Part model, mm, in its own coordinate system. A direction names the side the tool comes from. Round coordinates to 2 decimals unless told otherwise and drop trailing zeros. Write each loop counter-clockwise with the first axis right and the second up, starting at its lowest first coordinate (ties: lowest second). Pieces come first, ordered by that corner, then holes. Notation, with made-up numbers: M 63,23.25 L 78,23.25 A34 ccw 78,57.25 Z; hole C 70.5,36 d6. An arc over 180 degrees is marked long. Use a Markdown table: item, result. Add a question column.
1) Slice it at A-A on y = 16. Write the cut outline in (x, z), plus the area to 3 significant figures.
2) Drop flat-ended pins along their axis: P1, Ø0.9, axis at y = 17.5, z = 2, coming from the +X side; P2, Ø1.6, axis at x = -69.5, z = 2, coming from the -Y side; P3, Ø1.5, axis at y = 17.5, z = 1, coming from the -X side. Give the stop position or say it passes through.
3) Slice it at C-C on z = 1.8. Write the cut outline in (x, y), plus the area to 3 significant figures.
4) Which spindle directions (+Z, -Z, +X, -X, +Y, -Y) get a long thin tool onto all of the face, cutting with end or side? Do faces 4 (the face through (66.6, 21, 1)), 5 (the face through (66.6, -21, 1)), 6 (the face through (6, -20.5, 1)). Say none if no direction does.
5) Two-plate mould, pull along Y, no slides. Class faces 1 (the face through (-43.5, 0, 1)), 2 (the face through (65.17, -33.5, 1.48)), 3 (the face through (-66.6, 21, 1)): released by +Y, released by -Y, zero draft, split by the parting line, or undercut.
6) Slice it at D-D on x = 15.5. Write the cut outline in (y, z), plus the area to 3 significant figures.
7) Wall check: probe 1 along Y at (x, z) = (-40.7, 2.4); probe 2 along Y at (x, z) = (-19.5, 0.7); probe 3 along X at (y, z) = (28, 0.5). Give the ranges that are in metal, low to high.
8) Slice it at B-B on x = -40.7. Write the cut outline in (y, z).
```python
from build123d import *

# Parameters (mm, degrees)
ESQUISSE1_W                       = 101
ESQUISSE1_H                       = 41
BOSS_EXTRU_1_DEPTH                = 3
DIAM_TRE_DU_PER_AGE_3_0_3_1_D     = 3
DIAM_TRE_DU_PER_AGE_3_0_3_1_DEPTH = 3


with BuildPart() as part:
    # Esquisse1 → Boss.-Extru.1 (new body)
    with BuildSketch(Plane.XY):
        with BuildLine():
            Line((66.6, 30), (66.6, 12))
            ThreePointArc((66.6, 12), (67.185786438, 10.585786438), (68.6, 10))
            Line((68.6, 10), (70.6, 10))
            Line((70.6, 10), (70.6, -10))
            Line((70.6, -10), (68.6, -10))
            ThreePointArc((68.6, -10), (67.185786438, -10.585786438), (66.6, -12))
            Line((66.6, -12), (66.6, -30))
            ThreePointArc((66.6, -30), (65.135533906, -33.535533906), (61.6, -35))
            Line((61.6, -35), (-61.6, -35))
            ThreePointArc((-61.6, -35), (-65.135533906, -33.535533906), (-66.6, -30))
            Line((-66.6, -30), (-66.6, -12))
            ThreePointArc((-66.6, -12), (-67.185786438, -10.585786438), (-68.6, -10))
            Line((-68.6, -10), (-70.6, -10))
            Line((-70.6, -10), (-70.6, 10))
            Line((-70.6, 10), (-68.6, 10))
            ThreePointArc((-68.6, 10), (-67.185786438, 10.585786438), (-66.6, 12))
            Line((-66.6, 12), (-66.6, 30))
            ThreePointArc((-66.6, 30), (-65.135533906, 33.535533906), (-61.6, 35))
            Line((-61.6, 35), (61.6, 35))
            ThreePointArc((61.6, 35), (65.135533906, 33.535533906), (66.6, 30))
        make_face()
        with Locations((7, 0)):
            Rectangle(ESQUISSE1_W, ESQUISSE1_H, mode=Mode.SUBTRACT)
    extrude(amount=BOSS_EXTRU_1_DEPTH)

    # Diamètre du perçage Ø3.0 (3)1
    with Locations(Plane.XY.offset(3)):
        with Locations((-40.7, 27.7), (-40.7, -27.7), (54.7, -27.7), (54.7, 27.7)):
            Hole(DIAM_TRE_DU_PER_AGE_3_0_3_1_D / 2, depth=DIAM_TRE_DU_PER_AGE_3_0_3_1_DEPTH)


solid = part.part
```
Entries:
| question | item | result |
|---|---|---|
| 1 | outline | M -66.6,0 L -43.5,0 L -43.5,3 L -66.6,3 Z; M 57.5,0 L 66.6,0 L 66.6,3 L 57.5,3 Z |
| 1 | area | 96.6 mm^2 |
| 2 | P1 | stops at x = 66.6 |
| 2 | P2 | stops at y = -10 |
| 2 | P3 | stops at x = -66.6 |
| 3 | outline | M -70.6,-10 L -68.6,-10 A2 cw -66.6,-12 L -66.6,-30 A5 ccw -61.6,-35 L 61.6,-35 A5 ccw 66.6,-30 L 66.6,-12 A2 cw 68.6,-10 L 70.6,-10 L 70.6,10 L 68.6,10 A2 cw 66.6,12 L 66.6,30 A5 ccw 61.6,35 L -61.6,35 A5 ccw -66.6,30 L -66.6,12 A2 cw -68.6,10 L -70.6,10 Z; hole M -43.5,-20.5 L 57.5,-20.5 L 57.5,20.5 L -43.5,20.5 Z; hole C -40.7,-27.7 d3; hole C -40.7,27.7 d3; hole C 54.7,-27.7 d3; hole C 54.7,27.7 d3 |
| 3 | area | 5,300 mm^2 |
| 4 | face 4 | +Z, -Z, +X, +Y |
| 4 | face 5 | +Z, -Z, +X, -Y |
| 4 | face 6 | +Z, -Z |
| 5 | face 1 | undercut |
| 5 | face 2 | released by -Y |
| 5 | face 3 | zero draft |
| 6 | outline | M -35,0 L -20.5,0 L -20.5,3 L -35,3 Z; M 20.5,0 L 35,0 L 35,3 L 20.5,3 Z |
| 6 | area | 87.0 mm^2 |
| 7 | probe 1 | y = -35 to -29.2, -26.2 to -20.5, 20.5 to 26.2, 29.2 to 35 |
| 7 | probe 2 | y = -35 to -20.5, 20.5 to 35 |
| 7 | probe 3 | x = -66.6 to -42.17, -39.23 to 53.23, 56.17 to 66.6 |
| 8 | outline | M -35,0 L -29.2,0 L -29.2,3 L -35,3 Z; M -26.2,0 L -20.5,0 L -20.5,3 L -26.2,3 Z; M 20.5,0 L 26.2,0 L 26.2,3 L 20.5,3 Z; M 29.2,0 L 35,0 L 35,3 L 29.2,3 Z |
